Build history of the part. All positions in model axes, mm. A direction names the side the tool comes from. Give positions to 0.01 mm unless a question says otherwise; leave off trailing zeros. Write each loop counter-clockwise with the first axis right and the second up, starting at its lowest first coordinate (ties: lowest second). Pieces come first, ordered by that corner, then holes.
from build123d import *

# Parameters (mm, degrees)
PAD_DEPTH       = 6
THICKNESS_T     = -1.2
SKETCH001_R     = 2.6
POCKET_DEPTH    = 1.2
SKETCH002_R     = 2.6
POCKET001_DEPTH = 1.2
SKETCH003_R     = 2.6
POCKET002_DEPTH = 1.2


with BuildPart() as part:
    # Sketch → Pad (new body)
    with BuildSketch(Plane.XY):
        Polygon((80, -74), (65, -74), (-15, -22.5), (-85, -22.5), (-85, 22.5), (-15, 22.5), (15, 44), (30, 44), (30, 36), (15, 36), (-15, 14.5), (-15, 4), (0, 4), (0, -4), (-15, -4), (-15, -14.5), (65, -66), (80, -66), align=None)
    extrude(amount=PAD_DEPTH)

    # Thickness
    thickness_openings = [part.faces().sort_by_distance(p)[0] for p in [
        (-29.840547, -5.671982, 6),
    ]]
    offset(amount=THICKNESS_T, openings=thickness_openings, kind=Kind.INTERSECTION)

    # Sketch001 (on Face13 of Thickness) → Pocket (cut)
    with BuildSketch(Plane.YZ):
        with Locations((0, 6)):
            Circle(SKETCH001_R)
    extrude(amount=-POCKET_DEPTH, mode=Mode.SUBTRACT)

    # Sketch002 (on Face12 of Pocket) → Pocket001 (cut)
    with BuildSketch(Plane.YZ.offset(30)):
        with Locations((40, 6)):
            Circle(SKETCH002_R)
    extrude(amount=-POCKET001_DEPTH, mode=Mode.SUBTRACT)

    # Sketch003 (on Face2 of Pocket001) → Pocket002 (cut)
    with BuildSketch(Plane.YZ.offset(80)):
        with Locations((-70, 6)):
            Circle(SKETCH003_R)
    extrude(amount=-POCKET002_DEPTH, mode=Mode.SUBTRACT)


solid = part.part
1. Saw through at B-B on z = 5. Count the separate pieces of the cut face and the enclosed holes in it, plus the area to 3 significant figures.
2. Saw through at C-C on x = 3.5. Give the cut face in (y, z), plus the area to 3 significant figures.
3. Mould opens along X. For faces 5 (the face through (-16.2, -9, 4)), 6 (the face through (80, -70, 2)), 7 (the face through (-50, -22.5, 3)) say: pulls with the +X half, pulls with the -X half, needs draft (parallel to the pull), parting line crosses it, or undercut.
4. 3-axis set-ups, long thin cutter, end or side, ignore diameter. For faces 1 (the face through (23, 36, 3)), 2 (the face through (30, 40, 2)), 3 (the face through (-3, 24, 6)), 4 (the face through (-16.2, 9, 4)): which of +Z, -Z, +X, -X, +Y, -Y reach the whole face in a straight line?
5. Saw through at D-D on x = 35. Give the cut face in (y, z), plus the area to 3 significant figures.
6. Drill centre lines: line 1 along X through (y, z) = (-4.5, 3.25); line 2 along Y through (x, z) = (-24, 3.25); line 3 along Y through (x, z) = (-11, 5.5) (3 decimals). Where is each one in solid material? Low to high.
7. Drop flat-ended pins along their axis: pin 1 (2.5 mm diameter, centred on y = -70.5, z = 4.5, fed in from -X); pin 2 (3 mm diameter, centred on x = 59, z = 1, fed in from +Y); pin 3 (2.5 mm diameter, centred on x = -12.5, z = 2.5, fed in from -Y). Give the stop position or say it passes through.
8. Saw through at A-A on y = 0. Give the cut face in (x, z).
Outcome:
1. separate pieces: 3
1. enclosed holes: 0
1. area: 677 mm2
2. outline: (-34.41, 0) - (-26.41, 0) - (-26.41, 6) - (-27.84, 6) - (-27.84, 1.2) - (-32.98, 1.2) - (-32.98, 6) - (-34.41, 6) - close; (27.76, 0) - (35.76, 0) - (35.76, 6) - (34.28, 6) - (34.28, 1.2) - (29.23, 1.2) - (29.23, 6) - (27.76, 6) - close
2. area: 47.1 mm2
3. face 5: undercut
3. face 6: pulls with the +X half
3. face 7: needs draft
4. face 1: +Z, -Z, +X
4. face 2: +Z, -Z, +X, +Y
4. face 3: +Z, +X, -X, +Y, -Y
4. face 4: +Z
5. outline: (-54.69, 0) - (-46.69, 0) - (-46.69, 6) - (-48.11, 6) - (-48.11, 1.2) - (-53.26, 1.2) - (-53.26, 6) - (-54.69, 6) - close
5. area: 23.3 mm2
6. line 1: x = -85 to -83.8, -16.2 to -15
6. line 2: y = -22.5 to -21.3, 21.3 to 22.5
6. line 3: y = -25.075 to -23.648, -18.502 to -17.075, -4 to -2.8, 2.8 to 4, 17.367 to 18.843, 23.89 to 25.367
7. pin 1: stops at x = 57.62
7. pin 2: stops at y = -61.17
7. pin 3: stops at y = -24.91
8. outline: (-85, 0) - (0, 0) - (0, 3.4) - (-1.2, 3.4) - (-1.2, 1.2) - (-83.8, 1.2) - (-83.8, 6) - (-85, 6) - close
